Read the model definition and answer for the solid it produces. Units are mm, in the model's axes. Give positions to 0.01 mm unless a question says otherwise; leave off trailing zeros. Order: outer loops, then holes, each group sorted by start corner. A loop starts at its lowest first (then second) coordinate and runs counter-clockwise, first axis right, second up. Notation, with made-up numbers: (8.25, 21.25) -> (16.25, 21.25) arc R22 ccw to (16.25, 38.25) -> close; hole circle Ø9 at (35.5, 11). An arc over 180 degrees is marked (long way). Answer as CSV lines item,"result". Start each with the question number.
1) Find section C-C (z = 26). Determine the outline of the cut face in (x, y).
2) Straight lines are drawn through the part: L1, parallel to Z at x = 13, y = 324; L2, parallel to X at y = 461, z = 17.5; L3, parallel to Z at x = 20, y = 39.5. For each, find the intervals that lie inside material, in ascending order. Write a range as from..to.
3) Find section B-B (y = 736.6). Determine the outline of the cut face in (x, z), and give its area (3 significant figures).
4) Find section A-A (y = 239). Determine the outline of the cut face in (x, z), and give its area (3 significant figures).
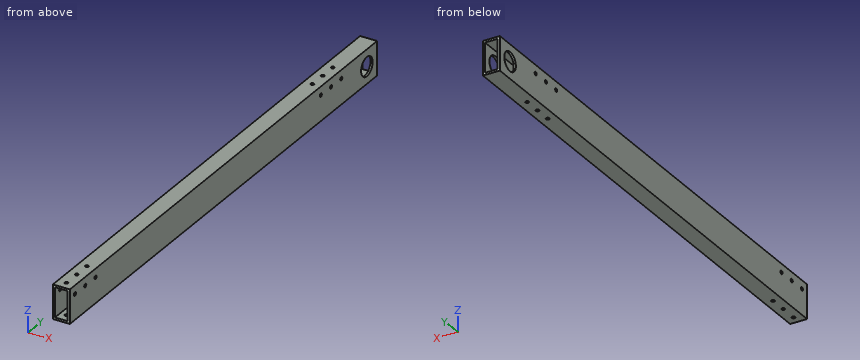
Autodesk Inventor part; units mm, degrees
ref_plane "YZ Plane" through (0, 0, 0) normal (1, 0, 0) x (0, 1, 0)
ref_plane "XZ Plane" through (0, 0, 0) normal (0, 1, 0) x (-1, 0, 0)
ref_plane "XY Plane" through (0, 0, 0) normal (0, 0, 1) x (1, 0, 0)
sketch "Sketch1" plane through (0, 0, 0) normal (0, 1, 0) x (-1, 0, 0)
  line L0 (2.2807, -2.5252) -> (-23.1193, -2.5252)
  line L1 (-23.1193, -2.5252) -> (-23.1193, 48.2748)
  line L2 (-23.1193, 48.2748) -> (2.2807, 48.2748)
  line L3 (2.2807, 48.2748) -> (2.2807, -2.5252)
  line L4 (-19.9443, 0.6498) -> (-0.8943, 0.6498)
  line L5 (-0.8943, 0.6498) -> (-0.8943, 45.0998)
  line L6 (-0.8943, 45.0998) -> (-19.9443, 45.0998)
  line L7 (-19.9443, 45.0998) -> (-19.9443, 0.6498)
  point P0 (0, 0)
  dimension "d0" = 25.4
  dimension "d1" = 50.8
  dimension "d2" = 3.175
extrude "Extrusion1" add sketch "Sketch1" along normal blind 762
sketch "Sketch3" plane through (-2.2807, 0, 48.2748) normal (0, 0, 1) x (1, 0, 0)
  line L0 (22.225, 0) -> (3.175, 0) construction
  line L1 (12.7, 0) -> (12.7, 12.7) construction
  line L2 (12.7, 12.7) -> (12.7, 38.1) construction
  line L3 (12.7, 38.1) -> (12.7, 63.5) construction
  circle A0 centre (12.7, 63.5) radius 2.5797
  circle A1 centre (12.7, 38.1) radius 2.5797
  circle A2 centre (12.7, 12.7) radius 2.5797
  line L4 (12.7, 685.8) -> (12.7, 673.1) construction
  circle A3 centre (12.7, 673.1) radius 2.5797
  line L5 (12.7, 673.1) -> (12.7, 647.7) construction
  line L6 (12.7, 647.7) -> (12.7, 622.3) construction
  circle A4 centre (12.7, 647.7) radius 2.5797
  circle A5 centre (12.7, 622.3) radius 2.5797
  point P0 (2.2807, 0)
  dimension "d19" = 12.7
  dimension "d20" = 25.4
  dimension "d21" = 25.4
  dimension "d22" = 5.1594
  dimension "d23" = 5.1594
  dimension "d24" = 5.1594
  dimension "d38" = 12.7
  dimension "d39" = 5.1594
  dimension "d40" = 25.4
  dimension "d41" = 25.4
  dimension "d42" = 5.1594
  dimension "d43" = 5.1594
extrude "Extrusion3" cut sketch "Sketch3" against normal blind 762
sketch "Sketch4" plane through (23.1193, 0, 48.2748) normal (1, 0, 0) x (0, 0, -1)
  line L0 (3.175, 762) -> (47.625, 762) construction
  line L1 (25.4, 762) -> (25.4, 736.6) construction
  point P0 (48.2748, 0)
  dimension "d44" = 25.4
sketch "Sketch5" plane through (-2.2807, 0, -2.5252) normal (-1, 0, 0) x (0, 0, 1)
  circle A0 centre (25.4, 12.7) radius 2.5797
  line L0 (50.8, 0) -> (50.8, 762)
  circle A1 centre (25.4, 38.1) radius 2.5797 construction
  line L1 (50.8, 38.1) -> (38.1, 38.1) construction
  circle A2 centre (25.4, 63.5) radius 2.5797 construction
  line L2 (50.8, 63.5) -> (38.1, 63.5) construction
  circle A3 centre (38.1, 63.5) radius 2.5797
  circle A4 centre (38.1, 38.1) radius 2.5797
  circle A5 centre (38.1, 12.7) radius 2.5797
  line L3 (38.1, 12.7) -> (50.8, 12.7) construction
  circle A6 centre (25.4, 622.3) radius 2.5797 construction
  line L4 (50.8, 622.3) -> (38.1, 622.3) construction
  circle A7 centre (25.4, 647.7) radius 2.5797 construction
  line L5 (50.8, 647.7) -> (38.1, 647.7) construction
  circle A8 centre (25.4, 673.1) radius 2.5797 construction
  line L6 (50.8, 673.1) -> (38.1, 673.1) construction
  circle A9 centre (38.1, 647.7) radius 2.5797
  circle A10 centre (38.1, 622.3) radius 2.5797
  circle A11 centre (38.1, 673.1) radius 2.5797
  point P0 (2.5252, 0)
  dimension "d46" = 12.7
  dimension "d47" = 12.7
  dimension "d48" = 5.1594
  dimension "d49" = 5.1594
  dimension "d50" = 5.1594
  dimension "d51" = 12.7
  dimension "d52" = 12.7
  dimension "d53" = 12.7
  dimension "d54" = 5.1594
  dimension "d55" = 5.1594
  dimension "d56" = 5.1594
extrude "Extrusion4" cut sketch "Sketch5" against normal blind 762 contours A3 | A4 | A5 | A9 | A10 | A11
sketch "Sketch6" plane through (-2.2807, 0, -2.5252) normal (-1, 0, 0) x (0, 0, 1)
  line L0 (47.625, 762) -> (3.175, 762) construction
  line L1 (25.4, 762) -> (25.4, 736.6) construction
  circle A0 centre (25.4, 736.6) radius 14.2875
  point P0 (2.5252, 0)
  dimension "d59" = 25.4
  dimension "d60" = 28.575
extrude "Extrusion5" cut sketch "Sketch6" against normal blind 304.8
properties part number "30in 1x1 Beam"
Findings below:
1,outline,"(-2.28, 0) -> (0.89, 0) -> (0.89, 722.66) -> (-2.28, 722.66) -> close; (-2.28, 750.54) -> (0.89, 750.54) -> (0.89, 762) -> (-2.28, 762) -> close; (19.94, 0) -> (23.12, 0) -> (23.12, 722.66) -> (19.94, 722.66) -> close; (19.94, 750.54) -> (23.12, 750.54) -> (23.12, 762) -> (19.94, 762) -> close"
2,L1,"-2.53..0.65, 45.1..48.27"
2,L2,"-2.28..0.89, 19.94..23.12"
2,L3,"-2.53..33.41, 37.74..48.27"
3,outline,"(-2.28, -2.53) -> (23.12, -2.53) -> (23.12, 8.59) -> (19.94, 8.59) -> (19.94, 0.65) -> (0.89, 0.65) -> (0.89, 8.59) -> (-2.28, 8.59) -> close; (-2.28, 37.16) -> (0.89, 37.16) -> (0.89, 45.1) -> (19.94, 45.1) -> (19.94, 37.16) -> (23.12, 37.16) -> (23.12, 48.27) -> (-2.28, 48.27) -> close"
3,area,"262 mm²"
4,outline,"(-2.28, -2.53) -> (23.12, -2.53) -> (23.12, 48.27) -> (-2.28, 48.27) -> close; hole (0.89, 0.65) -> (19.94, 0.65) -> (19.94, 45.1) -> (0.89, 45.1) -> close"
4,area,"444 mm²"
